Build history of the part. All positions in model axes, mm. Face numbers are marked on the shaded views. A direction names the side the tool comes from. Coordinates: 2 decimals unless noted, no trailing zeros. Write each loop counter-clockwise with the first axis right and the second up, starting at its lowest first coordinate (ties: lowest second). Pieces come first, ordered by that corner, then holes. Notation, with made-up numbers: M 0.5,28.25 L 46.5,28.25 A14 cw 46.5,43.25 Z; hole C 24.25,35.5 d1. An arc over 180 degrees is marked long. Use CSV: the item, a comma, the result in double quotes. Start each with the question number.
```python
from build123d import *

# Parameters (mm, degrees)
Y_KSEKLIK_EKSTR_ZYON1_DEPTH = 20.5
SKETCH_1_R                  = 2.5
EXTRUDE_1_DEPTH             = 2.5
SKETCH_2_R                  = 2.5
EXTRUDE_2_DEPTH             = 2.5
SKETCH_3_W                  = 20.5
SKETCH_3_H                  = 20.5
REVOLVE_2_ANGLE             = 90
SKETCH_4_R                  = 2.5
EXTRUDE_3_DEPTH             = 2.5


with BuildPart() as part:
    # Çizim1 → Yükseklik-Ekstrüzyon1 (new body)
    with BuildSketch(Plane.XY):
        with BuildLine():
            Line((0, 20.5), (0, 0))
            Line((0, 0), (20.5, 0))
            ThreePointArc((20.5, 0), (14.495689014, 14.495689014), (0, 20.5))
        make_face()
    extrude(amount=Y_KSEKLIK_EKSTR_ZYON1_DEPTH)

    # Эскиз1 → Бобышка-Вытянуть1 (add)
    with BuildSketch(Plane.ZY):
        with Locations(Location((10.25, 10.25, 0), (0, 0, 270))):
            Circle(SKETCH_1_R)
    extrude(amount=EXTRUDE_1_DEPTH)

    # Эскиз2 → Бобышка-Вытянуть2 (add)
    with BuildSketch(Plane(origin=(0, 0, 0), x_dir=(-1, 0, 0), z_dir=(0, -1, 0))):
        with Locations(Location((-10.25, -10.25, 0), (0, 0, 90))):
            Circle(SKETCH_2_R)
    extrude(amount=EXTRUDE_2_DEPTH)

    # Эскиз3 → Повернуть2 (revolve)
    with BuildSketch(Plane(origin=(0, 0, 0), x_dir=(-1, 0, 0), z_dir=(0, 0, -1))):
        with Locations((-10.25, 10.25)):
            Rectangle(SKETCH_3_W, SKETCH_3_H)
    revolve(axis=Axis((0, 0, 0), (1, 0, 0)), revolution_arc=REVOLVE_2_ANGLE)

    # Эскиз4 → Бобышка-Вытянуть3 (add)
    with BuildSketch(Plane(origin=(0, 0, 0), x_dir=(-1, 0, 0), z_dir=(0, 0, -1))):
        with Locations(Location((-10.25, 10.25, 0), (0, 0, 180))):
            Circle(SKETCH_4_R)
    extrude(amount=EXTRUDE_3_DEPTH)


solid = part.part
```
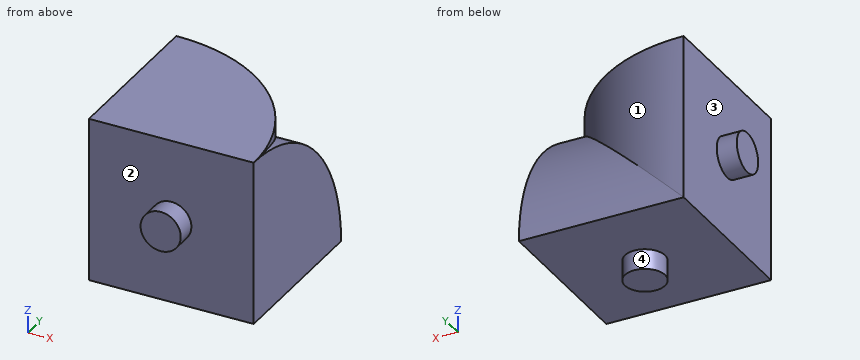
1. Slice it at B-B (y = 10.25). List the corners of the cut face in (x, z).
2. 3-axis set-ups, long thin cutter, end or side, ignore diameter. For the marked faces 1, 2, 3 and 4: which of +Z, -Z, +X, -X, +Y, -Y reach the whole face in a straight line?
3. Slice it at C-C (x = 10.25). List the corners of the cut face in (y, z), and give its area (3 significant figures).
4. Slice it at A-A (z = 8.5). List the corners of the cut face in (x, y).
5. Slice it at D-D (y = 2). List the corners of the cut face in (x, z).
6. Flat gauge pins, fed straight in: pin 1 (12 mm diameter, centred on x = 8.5, z = 16.5, fed in from +Y); pin 2 (1.5 mm diameter, centred on x = 16, z = 5.5, fed in from +Y); pin 3 (6 mm diameter, centred on y = 8.5, z = 0.5, fed in from -X). Where does each tip first touch, or does it go through?
7. Drill centre line: line 1 along Z through (x, y) = (3, 19). Where is it in solid material? Low to high. Write a range as from..to.
Established:
1,outline,"M -2.5,7.75 L 0,7.75 L 0,0 L 7.75,0 L 7.75,-2.5 L 12.75,-2.5 L 12.75,0 L 20.5,0 L 20.5,17.75 L 17.75,17.75 L 17.75,20.5 L 0,20.5 L 0,12.75 L -2.5,12.75 Z"
2,face 1,"+Z, +X, +Y"
2,face 2,"-Y"
2,face 3,"-X"
2,face 4,"-Z"
3,outline,"M -2.5,7.75 L 0,7.75 L 0,0 L 7.75,0 L 7.75,-2.5 L 12.75,-2.5 L 12.75,0 L 20.5,0 A20.5 ccw 17.75,10.25 L 17.75,20.5 L 0,20.5 L 0,12.75 L -2.5,12.75 Z"
3,area,"408 mm2"
4,outline,"M -2.5,8.46 L 0,8.46 L 0,0 L 8.46,0 L 8.46,-2.5 L 12.04,-2.5 L 12.04,0 L 20.5,0 L 20.5,18.65 L 8.5,18.65 A20.5 ccw 0,20.5 L 0,12.04 L -2.5,12.04 Z"
5,outline,"M 0,0 L 20.5,0 L 20.5,20.4 L 20.4,20.4 L 20.4,20.5 L 0,20.5 Z"
6,pin 1,"stops at y = 20.35"
6,pin 2,"stops at y = 19.94"
6,pin 3,"stops at x = 0"
7,line 1,"z = 0..20.5"
